```python
from build123d import *

# Parameters (mm, degrees)
SKETCH_6_W          = 42.3
SKETCH_6_H          = 42.3
SKETCH_6_R          = 1.6
SKETCH_6_R_2        = 15
EXTRUDE_1_DEPTH     = 5
SKETCH_7_R          = 1.6
SKETCH_7_R_2        = 4.15
EXTRUDE_5_DEPTH     = 38
SKETCH_7_7_R        = 4.15
SKETCH_7_7_R_2      = 1.6
EXTRUDE_7_DEPTH     = 38
SKETCH_7_8_R        = 4.15
SKETCH_7_8_R_2      = 1.6
EXTRUDE_8_DEPTH     = 38
SKETCH_12_W         = 2
SKETCH_12_H         = 44.3
EXTRUDE_11_DEPTH    = 38
SKETCH_14_W         = 44.3
SKETCH_14_H         = 2
EXTRUDE_12_DEPTH    = 38
SKETCH_15_W         = 2
SKETCH_15_H         = 42.3
EXTRUDE_13_DEPTH    = 38
CUT_EXTRUDE_1_DEPTH = 13.2
SKETCH_18_W         = 9.549489015
SKETCH_18_H         = 8.643215043
CUT_EXTRUDE_2_DEPTH = 123


with BuildPart() as part:
    # 草图6 → 凸台-拉伸1 (new body)
    with BuildSketch(Plane(origin=(0, 0, 0), x_dir=(1, 0, 0), z_dir=(0, 1, 0))):
        Rectangle(SKETCH_6_W, SKETCH_6_H)
        with Locations(Location((15.5, 15.5, 0), (0, 0, 270))):
            Circle(SKETCH_6_R, mode=Mode.SUBTRACT)
        with Locations(Location((-15.5, 15.5, 0), (0, 0, 270))):
            Circle(SKETCH_6_R, mode=Mode.SUBTRACT)
        with Locations(Location((-15.5, -15.5, 0), (0, 0, 270))):
            Circle(SKETCH_6_R, mode=Mode.SUBTRACT)
        with Locations(Location((15.5, -15.5, 0), (0, 0, 270))):
            Circle(SKETCH_6_R, mode=Mode.SUBTRACT)
        with Locations(Location((0, 0, 0), (0, 0, 270))):
            Circle(SKETCH_6_R_2, mode=Mode.SUBTRACT)
    extrude(amount=EXTRUDE_1_DEPTH)

    # 草图7 → 凸台-拉伸5 (add)
    with BuildSketch(Plane(origin=(0, 5, 0), x_dir=(1, 0, 0), z_dir=(0, 1, 0))):
        with BuildLine():
            Line((49, -79), (49, -64))
            ThreePointArc((49, -64), (48.724429591, -61.789948347), (47.914593709, -59.715235547))
            Line((47.914593709, -59.715235547), (21.15, -10.277072187))
            Line((21.15, -10.277072187), (21.15, -21.15))
            Line((21.15, -21.15), (10.070005019, -21.15))
            Line((10.070005019, -21.15), (30.963898233, -65.919418373))
            Line((30.963898233, -65.919418373), (30.963898233, -79))
            Line((30.963898233, -79), (49, -79))
        make_face()
        with Locations(Location((40, -76, 0), (0, 0, 270))):
            Circle(SKETCH_7_R, mode=Mode.SUBTRACT)
        with Locations(Location((40, -64, 0), (0, 0, 270))):
            Circle(SKETCH_7_R_2, mode=Mode.SUBTRACT)
        with BuildLine():
            Line((-30.963898233, -65.919418373), (-10.070005019, -21.15))
            Line((-10.070005019, -21.15), (-21.15, -21.15))
            Line((-21.15, -21.15), (-21.15, -10.282583808))
            Line((-21.15, -10.282583808), (-46.202269248, -57.478354795))
            ThreePointArc((-46.202269248, -57.478354795), (-48.271046585, -60.45179082), (-49, -64))
            Line((-49, -64), (-49, -79))
            Line((-49, -79), (-30.963898233, -79))
            Line((-30.963898233, -79), (-30.963898233, -65.919418373))
        make_face()
        with Locations(Location((-40, -76, 0), (0, 0, 270))):
            Circle(SKETCH_7_R, mode=Mode.SUBTRACT)
        with Locations(Location((-40, -64, 0), (0, 0, 270))):
            Circle(SKETCH_7_R_2, mode=Mode.SUBTRACT)
    extrude(amount=-EXTRUDE_5_DEPTH)


with BuildPart() as extrude_7_tool:
    # 草图7<7> → 凸台-拉伸7 (new body)
    with BuildSketch(Plane(origin=(0, 5, 0), x_dir=(1, 0, 0), z_dir=(0, 1, 0))):
        with Locations(Location((-40, -64, 0), (0, 0, 270))):
            Circle(SKETCH_7_7_R)
        with Locations(Location((40, -64, 0), (0, 0, 270))):
            Circle(SKETCH_7_7_R)
        with Locations(Location((40, -76, 0), (0, 0, 270))):
            Circle(SKETCH_7_7_R_2)
        with Locations(Location((-40, -76, 0), (0, 0, 270))):
            Circle(SKETCH_7_7_R_2)
    extrude(amount=EXTRUDE_7_DEPTH)


with BuildPart() as part_1:
    add(part.part)


with BuildPart() as part_2:
    # 凸台-拉伸7: joined with extrude_7_tool
    add(part_1.part.fuse(extrude_7_tool.part, tol=0.00001))


with BuildPart() as extrude_7_kept_piece:
    # of the separate pieces the step leaves, the one the design keeps (extrude_7_pieces_kept)
    add(part_2.part.solids().sort_by_distance((-10.070005019, 0, 21.15))[0])


with BuildPart() as extrude_8_tool:
    # 草图7<8> → 凸台-拉伸8 (new body)
    with BuildSketch(Plane(origin=(0, 5, 0), x_dir=(1, 0, 0), z_dir=(0, 1, 0))):
        with Locations(Location((-40, -64, 0), (0, 0, 270))):
            Circle(SKETCH_7_8_R)
        with Locations(Location((40, -64, 0), (0, 0, 270))):
            Circle(SKETCH_7_8_R)
        with Locations(Location((40, -76, 0), (0, 0, 270))):
            Circle(SKETCH_7_8_R_2)
        with Locations(Location((-40, -76, 0), (0, 0, 270))):
            Circle(SKETCH_7_8_R_2)
    extrude(amount=EXTRUDE_8_DEPTH)


with BuildPart() as extrude_7_kept_piece_1:
    add(extrude_7_kept_piece.part)


with BuildPart() as extrude_7_kept_piece_2:
    # 凸台-拉伸8: joined with extrude_8_tool
    add(extrude_7_kept_piece_1.part.fuse(extrude_8_tool.part, tol=0.00001))


with BuildPart() as extrude_8_kept_piece:
    # of the separate pieces the step leaves, the one the design keeps (extrude_8_pieces_kept)
    add(extrude_7_kept_piece_2.part.solids().sort_by_distance((-10.070005019, 0, 21.15))[0])

    # 草图12 → 凸台-拉伸11 (add)
    with BuildSketch(Plane(origin=(0, 5, 0), x_dir=(1, 0, 0), z_dir=(0, 1, 0))):
        with Locations((22.15, -1)):
            Rectangle(SKETCH_12_W, SKETCH_12_H)
    extrude(amount=-EXTRUDE_11_DEPTH)

    # 草图14 → 凸台-拉伸12 (add)
    with BuildSketch(Plane(origin=(0, 5, 0), x_dir=(1, 0, 0), z_dir=(0, 1, 0))):
        with Locations((-1, -22.15)):
            Rectangle(SKETCH_14_W, SKETCH_14_H)
    extrude(amount=-EXTRUDE_12_DEPTH)

    # 草图15 → 凸台-拉伸13 (add)
    with BuildSketch(Plane(origin=(0, 5, 0), x_dir=(1, 0, 0), z_dir=(0, 1, 0))):
        with Locations((-22.15, 0)):
            Rectangle(SKETCH_15_W, SKETCH_15_H)
    extrude(amount=-EXTRUDE_13_DEPTH)

    # 草图17 → 切除-拉伸1 (cut)
    with BuildSketch(Plane.XZ.offset(33)):
        Polygon((62.040525686, 30.953335803), (-8.604799232, 30.953335803), (-61.83718559, 30.953335803), (-61.83718559, 85.06296978), (-8.604799232, 85.06296978), (62.040525686, 85.06296978), align=None)
    extrude(amount=-CUT_EXTRUDE_1_DEPTH, mode=Mode.SUBTRACT)

    # 草图18 → 切除-拉伸2 (cut)
    with BuildSketch(Plane(origin=(49, 0, 0), x_dir=(0, 0, -1), z_dir=(1, 0, 0))):
        with Locations((-74.225255492, -8.321607522)):
            Rectangle(SKETCH_18_W, SKETCH_18_H)
    extrude(amount=-CUT_EXTRUDE_2_DEPTH, mode=Mode.SUBTRACT)


solid = extrude_8_kept_piece.part
```
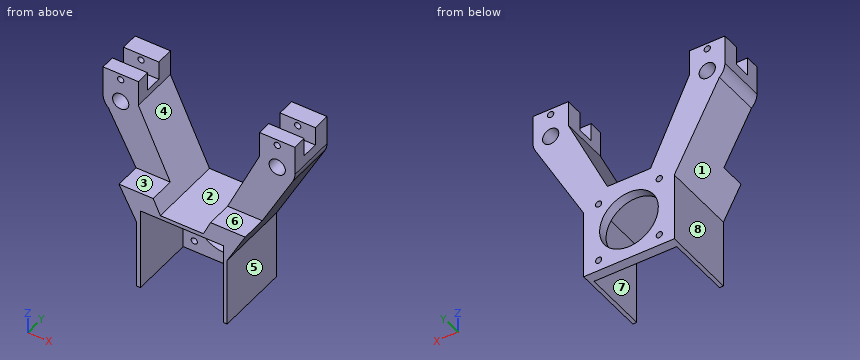
Model file for the job. Use its own axes, mm. Face numbers are marked on the shaded views. A direction names the side the tool comes from. Round coordinates to 2 decimals unless told otherwise and drop trailing zeros. Write each loop counter-clockwise with the first axis right and the second up, starting at its lowest first coordinate (ties: lowest second). Pieces come first, ordered by that corner, then holes. Notation, with made-up numbers: (-32.5, 39.5) - (-12.5, 39.5) arc R20 ccw to (-12.5, 76.5) - close; hole circle Ø3 at (-31.75, 47). An arc over 180 degrees is marked (long way). One line per item, written item: value.
(1) Wall check: probe 1 along X at (y, z) = (-17.25, 76); probe 2 along X at (y, z) = (1.85, -15.5); probe 3 along X at (y, z) = (-24, 4). Give the ranges that are in metal, low to high.
Values follow:
probe 1: x = -49 to -41.6, -38.4 to -30.96, 30.96 to 38.4, 41.6 to 49
probe 2: x = -23.15 to -17.1, -13.9 to 13.9, 17.1 to 23.15
probe 3: x = -23.15 to -21.15, 21.15 to 23.15
(2) 3-axis set-ups, long thin cutter, end or side, ignore diameter. For the marked faces 5, 6, 7 and 8: which of +Z, -Z, +X, -X, +Y, -Y reach the whole face in a straight line?
Values follow:
face 5: -Z, +X, +Y, -Y
face 6: +Z, +X, -X, -Y
face 7: -Z, -Y
face 8: -Z, -X, +Y, -Y
(3) Cut at D-D, the plane z = 26. Give the cut face in (x, y), plus the area to 3 significant figures.
Values follow:
outline: (-29.49, -33) - (-12.33, -33) - (-12.33, 5) - (-29.49, 5) - close; (12.33, -33) - (29.66, -33) - (29.66, 5) - (12.33, 5) - close
area: 1,310 mm²
(4) Drop flat-ended pins along their axis: P1, Ø2.5, axis at x = -42, y = -9, coming from the +Z side; P2, Ø8, axis at x = 36, y = -26.5, coming from the -Z side; P3, Ø12, axis at y = -16, z = 44, coming from the +X side (3 decimals). Give the stop position or say it passes through.
Values follow:
P1: stops at z = 69.45
P2: stops at z = 30.32
P3: stops at x = 42.655
(5) Two-plate mould, pull along X, no slides. Class the marked faces 1, 2, 3 and 4: pulls with the +X half, pulls with the -X half, needs draft (parallel to the pull), parting line crosses it, or undercut.
Values follow:
face 1: pulls with the -X half
face 2: undercut
face 3: needs draft
face 4: undercut
(6) Cut at B-B, the plane x = 0. Give the cut face in (y, z), plus the area to 4 significant figures.
Values follow:
outline: (-33, 21.15) - (0, 21.15) - (0, 15) - (5, 15) - (5, 23.15) - (-33, 23.15) - close; (0, -21.15) - (5, -21.15) - (5, -15) - (0, -15) - close
area: 137.5 mm²
(7) Cut at A-A, the plane z = 76. Give the number of separate pieces and of enclosed holes in the cut face, plus the area to 3 significant figures.
Values follow:
separate pieces: 8
enclosed holes: 0
area: 479 mm²
